```python
from build123d import *

# Parameters (mm, degrees)
F0_R     = 2.1
F0_R_2   = 1.3
F1_DEPTH = 15
F0_R_3   = 2.85
F2_DEPTH = 7
F0_R_4   = 4
F3_DEPTH = 8
F5_R     = 0.8


# Not quite as in the source:
# - a fillet or chamfer that OpenCascade refuses, or shapes differently, is made with other operations: its cross-section is extruded or revolved along the edge and cut away or added


with BuildPart() as f1:
    # F0 (on Top) → F1 (new body)
    with BuildSketch(Plane.XY):
        Circle(F0_R)
        Circle(F0_R_2, mode=Mode.SUBTRACT)
    extrude(amount=F1_DEPTH)

    # F0 (on Top) → F2 (join)
    with BuildSketch(Plane.XY):
        Circle(F0_R_3)
        Circle(F0_R, mode=Mode.SUBTRACT)
        Circle(F0_R)
        Circle(F0_R_2, mode=Mode.SUBTRACT)
    extrude(amount=-F2_DEPTH)

    # F0 (on Top) → F3 (join)
    with BuildSketch(Plane.XY):
        Circle(F0_R_4)
        Circle(F0_R_3, mode=Mode.SUBTRACT)
        Circle(F0_R_3)
        Circle(F0_R, mode=Mode.SUBTRACT)
    extrude(amount=F3_DEPTH)

    # F4: fillet of radius 2.3 on 1 edges, made by hand

    # F4_s1 → F4_t2 (revolve, cut)
    with BuildSketch(Plane.XZ):
        with BuildLine():
            ThreePointArc((2.1, 8), (3.4621010187, 7.2132242193), (4, 5.7350496694))
            Line((4, 5.7350496694), (4, 8))
            Line((4, 8), (2.1, 8))
        make_face()
    revolve(axis=Axis((0, 0, 8), (0, 0, 1)), mode=Mode.SUBTRACT)

    # F5
    f5_edges = [f1.edges().sort_by_distance(p)[0] for p in [
        (-2.85, 0, -7),
    ]]
    fillet(f5_edges, radius=F5_R)


solid = f1.part
```
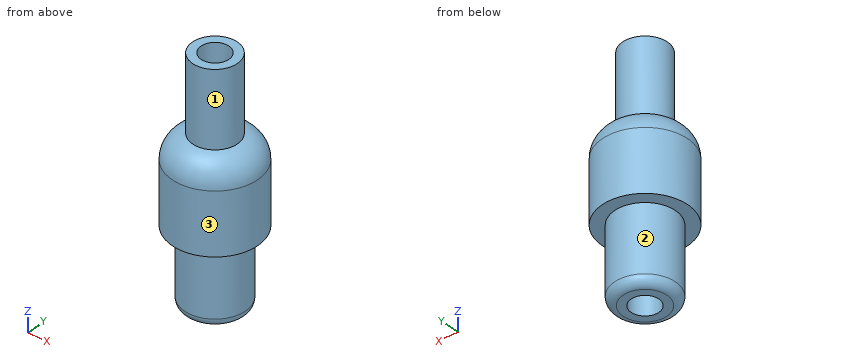
Work out the finished part from the listing and answer in its coordinate system (mm). Face numbers are marked on the shaded views. A direction names the side the tool comes from. Coordinates: 2 decimals unless noted, no trailing zeros. Loops run counter-clockwise (first coordinate to the right, second up) from the corner with the lowest first, then second, coordinate; pieces in that order, holes last. Notation, with made-up numbers: (79, 38) - (110, 38) arc R10 cw to (110, 44) - close; hole circle Ø7 at (38.25, 7.25). An arc over 180 degrees is marked (long way). Use a Markdown table: item, result.
Item 1: Find section A-A, the plane z = 9.75. Determine the outline of the cut face in (x, y), and give its area (3 significant figures).
Evaluation:
| item | result |
|---|---|
| outline | circle Ø4.2 at (0, 0); hole circle Ø2.6 at (0, 0) |
| area | 8.55 mm2 |
Item 2: Consider probe 1 along Y at (x, z) = (0, 11.25); probe 2 along Y at (x, z) = (0, -3.5); probe 3 along X at (y, z) = (0.5, -2.5). Determine where each line is inside the solid, lowest interval first. Write a range as from..to.
Evaluation:
| item | result |
|---|---|
| probe 1 | y = -2.1..-1.3, 1.3..2.1 |
| probe 2 | y = -2.85..-1.3, 1.3..2.85 |
| probe 3 | x = -2.81..-1.2, 1.2..2.81 |
Item 3: Given pin 1 Ø3.5 at (x, y) = (0, 0) entering from +Z; pin 2 Ø1 at (x, z) = (2.5, -3) entering from -Y; pin 3 Ø4 at (x, z) = (-0.5, -3.5) entering from +Y; pin 4 Ø1 at (x, z) = (3, 0) entering from +Y, each flat-ended and moving along its own axis, determine where each tip first touches the part or whether it passes through.
Evaluation:
| item | result |
|---|---|
| pin 1 | stops at z = 15 |
| pin 2 | stops at y = -2.03 |
| pin 3 | stops at y = 2.85 |
| pin 4 | stops at y = 3.12 |
Item 4: Find section B-B, the plane z = -2.75. Determine the outline of the cut face in (x, y).
Evaluation:
| item | result |
|---|---|
| outline | circle Ø5.7 at (0, 0); hole circle Ø2.6 at (0, 0) |
Item 5: For the marked faces 1, 2 and 3, determine the directions among +Z, -Z, +X, -X, +Y, -Y from which every point of the face is accessible in a straight line to the end or side of a thin tool.
Evaluation:
| item | result |
|---|---|
| face 1 | +Z |
| face 2 | -Z |
| face 3 | +Z, -Z |
